```python
from build123d import *

# Parameters (mm, degrees)
FSHAPE1_DEPTH    = 20
FRSHAPE1_R       = 10
FPIN1ABASE_REACH = 23
SPIN1ABASE_R     = 5
FPIN1BBASE_REACH = 23
SPIN1BBASE_R     = 5
FPIN2BASE_REACH  = 23
SPIN2BASE_R      = 5


with BuildPart() as part:
    # SShape1 → FShape1 (new body)
    with BuildSketch(Plane(origin=(0, 1, 0), x_dir=(1, 0, 0), z_dir=(0, 1, 0))):
        Polygon((-15, 25), (15, 25), (27.5, -25), (-27.5, -25), align=None)
    extrude(amount=FSHAPE1_DEPTH)

    # FRShape1
    frshape1_edges = [part.edges().sort_by_distance(p)[0] for p in [
        (-15, 11, -25),
        (15, 11, -25),
        (27.5, 11, 25),
        (-27.5, 11, 25),
    ]]
    fillet(frshape1_edges, radius=FRSHAPE1_R)

    # SPin1aBase → FPin1aBase (add, up to next)
    with BuildSketch(Plane(origin=(0, 0, 0), x_dir=(1, 0, 0), z_dir=(0, 1, 0)), mode=Mode.PRIVATE) as fpin1abase_sk1:
        with Locations((6.84160069, -3.95)):
            Circle(SPIN1ABASE_R)
    fpin1abase_tool1 = extrude(fpin1abase_sk1.sketch, amount=FPIN1ABASE_REACH, mode=Mode.PRIVATE) - part.part
    add(fpin1abase_tool1.solids().sort_by_distance((6.841601, 0, 3.95))[0])

    # SPin1bBase → FPin1bBase (add, up to next)
    with BuildSketch(Plane(origin=(0, 0, 0), x_dir=(1, 0, 0), z_dir=(0, 1, 0)), mode=Mode.PRIVATE) as fpin1bbase_sk1:
        with Locations((-6.84160069, -3.95)):
            Circle(SPIN1BBASE_R)
    fpin1bbase_tool1 = extrude(fpin1bbase_sk1.sketch, amount=FPIN1BBASE_REACH, mode=Mode.PRIVATE) - part.part
    add(fpin1bbase_tool1.solids().sort_by_distance((-6.841601, 0, 3.95))[0])

    # SPin2Base → FPin2Base (add, up to next)
    with BuildSketch(Plane(origin=(0, 0, 0), x_dir=(1, 0, 0), z_dir=(0, 1, 0)), mode=Mode.PRIVATE) as fpin2base_sk1:
        with Locations((0, 10.3)):
            Circle(SPIN2BASE_R)
    fpin2base_tool1 = extrude(fpin2base_sk1.sketch, amount=FPIN2BASE_REACH, mode=Mode.PRIVATE) - part.part
    add(fpin2base_tool1.solids().sort_by_distance((0, 0, -10.3))[0])


solid = part.part
```
For this review, take the finished solid that the model builds, in its own axes (mm). A direction names the side the tool comes from. Round coordinates to 2 decimals unless told otherwise and drop trailing zeros. Write each loop counter-clockwise with the first axis right and the second up, starting at its lowest first coordinate (ties: lowest second). Pieces come first, ordered by that corner, then holes.
1) Take a section at D-D on z = 5. Give the boundary of the cut face in (x, y), then the cut area to 3 significant figures.
Answer below:
outline: (-22.5, 1) - (-11.73, 1) - (-11.73, 0) - (-1.95, 0) - (-1.95, 1) - (1.95, 1) - (1.95, 0) - (11.73, 0) - (11.73, 1) - (22.5, 1) - (22.5, 21) - (-22.5, 21) - close
area: 920 mm2
2) Mouldability with a two-part tool opening along X and no side actions: class faces 3 (the face through (0, 0, -10)), 4 (the face through (2.87, 0.49, 6.99)), 5 (the face through (-20.7, 10.9, -2.2)) as +X half, -X half, draft (parallel to the pull), parting line (faces both ways), or undercut.
Answer below:
face 3: draft
face 4: undercut
face 5: -X half
3) Machinability: for faces 1 (the face through (-7, 0, 4)), 2 (the face through (-2.223, 0.493, 5.865)), which of the approach directions +Z, -Z, +X, -X, +Y, -Y give a long, thin tool a straight path to every point of the face, cutting with its end or side? Answer none if there is none.
Answer below:
face 1: +Z, -Z, +X, -X, -Y
face 2: -Y
4) Insertion check: pin 1 Ø3 at (x, y) = (18, 9.5) entering from +Z; pin 2 Ø1 at (y, z) = (5, 17) entering from +X; pin 3 Ø1.5 at (x, z) = (11.5, 10) entering from -Y. Each pin has a flat end and moves straight along its axis. Give the tip position at first contact, or say it passes through.
Answer below:
pin 1: stops at z = 24.84
pin 2: stops at x = 24.58
pin 3: stops at y = 1
5) Take a section at A-A on x = 0. Give the boundary of the cut face in (y, z), then the cut area to 3 significant figures.
Answer below:
outline: (0, -15.3) - (1, -15.3) - (1, -25) - (21, -25) - (21, 25) - (1, 25) - (1, -5.3) - (0, -5.3) - close
area: 1,010 mm2
6) For line 1 along Y through (x, z) = (-13.5, -22); line 2 along Z through (x, y) = (7.5, 6.75); line 3 along X through (y, z) = (11.75, -0.5) (3 decimals), list the stretches that pass through material, from the lowest coordinate up.
Answer below:
line 1: y = 1 to 21
line 2: z = -25 to 25
line 3: x = -21.125 to 21.125
7) Take a section at B-B on z = -10.3. Give the boundary of the cut face in (x, y) (3 decimals).
Answer below:
outline: (-18.675, 1) - (-5, 1) - (-5, 0) - (5, 0) - (5, 1) - (18.675, 1) - (18.675, 21) - (-18.675, 21) - close
8) Take a section at C-C on z = -4. Give the boundary of the cut face in (x, y), then the cut area to 3 significant figures.
Answer below:
outline: (-20.25, 1) - (20.25, 1) - (20.25, 21) - (-20.25, 21) - close
area: 810 mm2
